from build123d import *

# Parameters (mm, degrees)
SKETCH1_W                    = 304.8
SKETCH1_H                    = 1.5875
BASE_FLANGE1_DEPTH           = 50.8
EDGE_FLANGE1_STRIP_W         = 16.51
EDGE_FLANGE1_STRIP_H         = 1.5875
EDGE_FLANGE1_STRIP_CUT_DEPTH = 304.8
EDGE_FLANGE1_DEPTH           = 304.8
SKETCH10_R                   = 2.38125
CUT_EXTRUDE1_DEPTH           = 163.199630568
FILLET1_R                    = 12


# Sheet-metal steps are written as plain solids
with BuildPart() as part:
    # Sketch1 → Base-Flange1 (new body)
    with BuildSketch(Plane(origin=(0, 0, 0), x_dir=(1, 0, 0), z_dir=(0, 1, 0))):
        with Locations((0, -0.79375)):
            Rectangle(SKETCH1_W, SKETCH1_H)
    extrude(amount=BASE_FLANGE1_DEPTH)

    # Edge-Flange1 strip (across the edge) → Edge-Flange1 strip cut (cut)
    with BuildSketch(Plane(origin=(152.4, 50.8, 1.5875), x_dir=(0, -1, 0), z_dir=(-1, 0, 0))):
        with Locations((-1.5875, -0.79375)):
            Rectangle(EDGE_FLANGE1_STRIP_W, EDGE_FLANGE1_STRIP_H)
    extrude(amount=EDGE_FLANGE1_STRIP_CUT_DEPTH, mode=Mode.SUBTRACT)

    # Edge-Flange1 section (across the edge) → Edge-Flange1 (add)
    with BuildSketch(Plane(origin=(152.4, 50.8, 1.5875), x_dir=(0, -1, 0), z_dir=(-1, 0, 0))):
        with BuildLine():
            Line((0, 5.08), (0, 22.4125))
            Line((0, 22.4125), (1.5875, 22.4125))
            Line((1.5875, 22.4125), (1.5875, 5.08))
            ThreePointArc((1.5875, 5.08), (3.075397552, 1.487897552), (6.6675, 0))
            Line((6.6675, 0), (6.6675, -1.5875))
            ThreePointArc((6.6675, -1.5875), (1.952865536, 0.365365536), (0, 5.08))
        make_face()
    extrude(amount=EDGE_FLANGE1_DEPTH)

    # Sketch10 → Cut-Extrude1 (cut, through all)
    with BuildSketch(Plane.XY.offset(1.5875)):
        with Locations((-114.3, 19.05)):
            Circle(SKETCH10_R)
        with Locations((114.3, 19.05)):
            Circle(SKETCH10_R)
        with Locations((0, 19.05)):
            Circle(SKETCH10_R)
        with Locations((57.15, 19.05)):
            Circle(SKETCH10_R)
        with Locations((-57.15, 19.05)):
            Circle(SKETCH10_R)
    extrude(amount=-CUT_EXTRUDE1_DEPTH, mode=Mode.SUBTRACT)

    # Fillet1
    fillet1_edges = [part.edges().sort_by_distance(p)[0] for p in [
        (152.4, 50.00625, 24),
        (-152.4, 50.00625, 24),
        (-152.4, 0, 0.79375),
        (152.4, 0, 0.79375),
    ]]
    fillet(fillet1_edges, radius=FILLET1_R)


solid = part.part
Input: part model. Units: mm. Frame: model coordinates. A direction names the side the tool comes from. Round coordinates to 2 decimals unless told otherwise and drop trailing zeros. Loops run counter-clockwise (first coordinate to the right, second up) from the corner with the lowest first, then second, coordinate; pieces in that order, holes last. Notation, with made-up numbers: (-10, 84.25) -> (36, 84.25) arc R27 ccw to (36, 114.25) -> close; hole circle Ø1 at (16.25, -21.5). An arc over 180 degrees is marked (long way). Answer as a JSON object with one key per item and string values. Group by question number.
1) Section query B-B on y = 33. Output: boundary loops of the cut face in (x, z).
2) Pin query (flat end, axial travel): pin 1 (2 mm diameter, centred on x = -60, z = 15.5, fed in from -Y); pin 2 (6 mm diameter, centred on x = -114.3, y = 19.05, fed in from +Z); pin 3 (4 mm diameter, centred on x = 57.15, y = 19.05, fed in from +Z); pin 4 (7.5 mm diameter, centred on x = 0, y = 19.05, fed in from -Z). Return the tip coordinate at first contact, or that it passes through.
3) Section query A-A on x = -22. Output: boundary loops of the cut face in (y, z) (1 decimal), plus the area to 3 significant figures.
4) Reachability of faces 4 (the flat face through (-152.4, 34, 1)), 5 (the flat face through (2, 49.212, 15)) from +Z, -Z, +X, -X, +Y, -Y: full face, straight path, thin tool, end or side. Return the list, or none.
5) Ray query, L1, parallel to Z at x = 91, y = 37; L2, parallel to Y at x = 101.5, z = 8.75; L3, parallel to Y at x = 57.15, z = 0.5. Return the intervals inside material, ascending.
6) Section query C-C on z = 17.25. Output: boundary loops of the cut face in (x, y), plus the area to 3 significant figures.
7) Draft query along Y for faces 1 (the cylindrical face through (1.1, 16.94, 0.8)), 2 (the cylindrical face through (-148.79, 50, 20.58)), 3 (the cylindrical face through (148.98, 3.61, 0.78)). Return one class per face: +Y half, -Y half, draft (parallel to the pull), parting line (faces both ways), or undercut.
Reply:
{
 "1": {"outline": "(-152.4, 0) -> (152.4, 0) -> (152.4, 1.59) -> (-152.4, 1.59) -> close"},
 "2": {"pin 1": "stops at y = 49.21", "pin 2": "stops at z = 1.59", "pin 3": "passes through", "pin 4": "stops at z = 0"},
 "3": {"outline": "(0, 0) -> (44.1, 0) arc R6.7 ccw to (50.8, 6.7) -> (50.8, 24) -> (49.2, 24) -> (49.2, 6.7) arc R5.1 cw to (44.1, 1.6) -> (0, 1.6) -> close", "area": "112 mm2"},
 "4": {"face 4": "+Z, -Z, -X, +Y, -Y", "face 5": "+Z, +X, -X, -Y"},
 "5": {"L1": "z = 0 to 1.59", "L2": "y = 49.21 to 50.8", "L3": "y = 0 to 16.67, 21.43 to 46.67"},
 "6": {"outline": "(-151.19, 49.21) -> (151.19, 49.21) -> (151.19, 50.8) -> (-151.19, 50.8) -> close", "area": "480 mm2"},
 "7": {"face 1": "undercut", "face 2": "draft", "face 3": "-Y half"}
}
